For this review, take the finished solid that the model builds, in its own axes (mm). Face numbers are marked on the shaded views. A direction names the side the tool comes from. Coordinates: 2 decimals unless noted, no trailing zeros. Loops run counter-clockwise (first coordinate to the right, second up) from the corner with the lowest first, then second, coordinate; pieces in that order, holes last. Notation, with made-up numbers: M -13,20 L 23,20 A27 cw 23,53 Z; hole C -7.75,37.25 d10. An arc over 180 degrees is marked long. Write item = value, one per line.
from build123d import *

# Parameters (mm, degrees)
PAD_DEPTH       = 6
SKETCH001_R     = 3
POCKET_DEPTH    = 6.001
SKETCH002_W     = 5.4
SKETCH002_H     = 2.5
POCKET001_DEPTH = 150.72142


with BuildPart() as part:
    # Sketch → Pad (new body)
    with BuildSketch(Plane.YZ):
        Polygon((-20, -30), (-20, 30), (-10, 30), (-10, 24), (10, 24), (10, 30), (20, 30), (20, -30), (10, -30), (10, -24), (-10, -24), (-10, -30), align=None)
    extrude(amount=PAD_DEPTH)

    # Sketch001 (on Face14 of Pad) → Pocket (cut, through all)
    with BuildSketch(Plane.YZ.offset(6)):
        with Locations((0, 10)):
            Circle(SKETCH001_R)
    extrude(amount=-POCKET_DEPTH, mode=Mode.SUBTRACT)

    # Sketch002 (on Face5 of Pocket) → Pocket001 (cut, through all)
    with BuildSketch(Plane.YZ.offset(6)):
        with Locations((0, 19.75)):
            Rectangle(SKETCH002_W, SKETCH002_H)
    pocket001 = extrude(amount=-POCKET001_DEPTH, mode=Mode.SUBTRACT)

    # Mirrored: Pocket001 across Sketch002 H_Axis
    add(pocket001.mirror(Plane(origin=(6, 0, 0), x_dir=(1, 0, 0), z_dir=(0, 0, 1))), mode=Mode.SUBTRACT)


solid = part.part
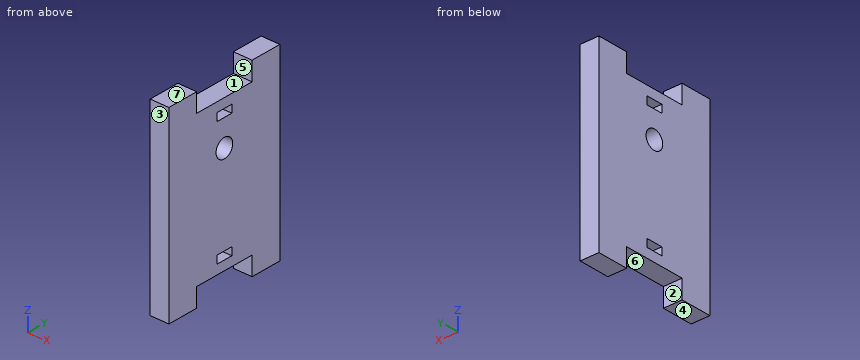
Q1. Add section D-D (y = 8.5). Write out the cut boundary in (x, z).
Solved:
outline = M 0,-24 L 6,-24 L 6,24 L 0,24 Z
Q2. Add section B-B (y = 0). Write out the cut boundary in (x, z), and give its area (3 significant figures).
Solved:
outline = M 0,-24 L 6,-24 L 6,-21 L 0,-21 Z; M 0,-18.5 L 6,-18.5 L 6,7 L 0,7 Z; M 0,13 L 6,13 L 6,18.5 L 0,18.5 Z; M 0,21 L 6,21 L 6,24 L 0,24 Z
area = 222 mm²
Q3. Add section C-C (x = 1.2). Write out the cut boundary in (y, z), and give its area (3 significant figures).
Solved:
outline = M -20,-30 L -10,-30 L -10,-24 L 10,-24 L 10,-30 L 20,-30 L 20,30 L 10,30 L 10,24 L -10,24 L -10,30 L -20,30 Z; hole C 0,10 d6; hole M -2.7,-21 L 2.7,-21 L 2.7,-18.5 L -2.7,-18.5 Z; hole M -2.7,18.5 L 2.7,18.5 L 2.7,21 L -2.7,21 Z
area = 2,100 mm²
Q4. Add section A-A (z = 10). Write out the cut boundary in (x, y).
Solved:
outline = M 0,-20 L 6,-20 L 6,-3 L 0,-3 Z; M 0,3 L 6,3 L 6,20 L 0,20 Z
Q5. For line 1 along Z through (x, y) = (2.9, 0); line 2 along Y through (x, z) = (0.95, -26.5); line 3 along Y through (x, z) = (0.85, -20.5), list the stretches that pass through material, from the lowest coordinate up.
Solved:
line_1 = -24 to -21, -18.5 to 7, 13 to 18.5, 21 to 24
line_2 = -20 to -10, 10 to 20
line_3 = -20 to -2.7, 2.7 to 20
Q6. Draft analysis for pull direction Y (two halves, no side actions). For the marked faces 1, 2, 3 and 4, state which applies: +Y half, -Y half, draft (parallel to the pull), parting line (faces both ways), or undercut.
Solved:
face_1 = undercut
face_2 = undercut
face_3 = -Y half
face_4 = draft
Q7. Machinability: for the marked faces 5, 6 and 7, which of the approach directions +Z, -Z, +X, -X, +Y, -Y give a long, thin tool a straight path to every point of the face, cutting with its end or side? Answer none if there is none.
Solved:
face_5 = +Z, +X, -X
face_6 = -Z, +X, -X
face_7 = +Z, +X, -X, +Y, -Y
Q8. For pin 1 Ø1.6 at (x, y) = (2, -1) entering from -Z; pin 2 Ø1.8 at (x, y) = (3.5, 0) entering from +Z, all flat-tipped, find the tip position at first contact; note any pin that passes through.
Solved:
pin_1 = -24
pin_2 = 24
